Part model, mm, in its own coordinate system. A direction names the side the tool comes from. Round coordinates to 2 decimals unless told otherwise and drop trailing zeros. Order: outer loops, then holes, each group sorted by start corner. A loop starts at its lowest first (then second) coordinate and runs counter-clockwise, first axis right, second up. Notation, with made-up numbers: M 26.5,-4 L 59.5,-4 A36 ccw 59.5,31 Z; hole C -39,20 d7. An arc over 180 degrees is marked long. Write each question's results on one line, items separated by ' | '. Start each with the question number.
1. Band-saw the part on A-A, the plane x = 49. List the corners of the cut face in (y, z).
2. Drop flat-ended pins along their axis: pin 1 Ø8 at (x, z) = (38, 71) entering from +Y; pin 2 Ø1 at (x, y) = (24, -1.5) entering from -Z. Give the stop position or say it passes through.
3. Band-saw the part on D-D, the plane z = 35. List the corners of the cut face in (x, y), then the cut area to 3 significant figures.
4. Band-saw the part on C-C, the plane x = 19. List the corners of the cut face in (y, z), then the cut area to 3 significant figures.
5. Band-saw the part on B-B, the plane z = 19. List the corners of the cut face in (x, y), then the cut area to 3 significant figures.
6. Which spindle directions (+Z, -Z, +X, -X, +Y, -Y) get a long thin tool onto all of the face, cutting with end or side? Do faces 1 (the face through (26.538, 0.371, 111.632)), 2 (the face through (27.28, 0.33, 110.64)). Say none if no direction does.
7. Probe L1, parallel to Z at x = 31.5, y = -1.35; L2, parallel to Y at x = 38, z = 47.5; L3, parallel to Z at x = 14, y = -0.85. List the from-to ranges inside material, lowest first. Write a range as [from, to].
Autodesk Inventor part; units mm, degrees
ref_plane "YZ Plane" through (0, 0, 0) normal (1, 0, 0) x (0, 1, 0)
ref_plane "XZ Plane" through (0, 0, 0) normal (0, 1, 0) x (-1, 0, 0)
ref_plane "XY Plane" through (0, 0, 0) normal (0, 0, 1) x (1, 0, 0)
sketch "Sketch1" plane through (0, 0, 0) normal (0, 0, 1) x (1, 0, 0)
  line L0 (0.222, 0) -> (0.222, -1)
  line L1 (0.222, 0) -> (0.222, -5.0532)
  line L2 (0.222, -1) -> (-0.778, -1)
  line L3 (-0.778, -1) -> (-0.778, -2.2)
  line L4 (53.594, 0) -> (55.372, 0)
  line L5 (53.594, 0) -> (53.594, -1)
  line L6 (53.594, 0) -> (53.594, -17.7031)
  line L7 (53.594, -1) -> (54.594, -1)
  line L8 (54.594, -1) -> (54.594, -2.2)
  line L9 (-1.778, 0) -> (-1.778, -17.5378)
  line L10 (-0.778, -2.2) -> (54.594, -2.2)
  line L11 (0.222, 0) -> (53.372, 0)
  line L12 (0.222, -1) -> (53.594, -1)
  line L13 (-0.778, -2.2) -> (54.594, -2.2)
  line L14 (54.594, -2.2) -> (54.594, -1)
  line L15 (54.594, -1) -> (-0.778, -1)
  line L16 (-0.778, -1) -> (-0.778, -2.2)
  line L17 (-0.278, -2.2) -> (-0.278, -1)
  line L18 (54.094, -2.2) -> (54.094, -1)
  point P0 (0, 0)
  point P1 (26.797, 5.3109)
  dimension "d0" = 1
  dimension "d1" = 1
  dimension "d2" = 1.2
  dimension "d3" = 1
  dimension "d4" = 1
  dimension "d5" = 1.2
extrude "Extrusion1" add sketch "Sketch1" along normal blind 111.76 contours L12 L6 L10 L1 | L1 L10 L17 L2 | L7 L18 L10 L6
sketch "Sketch2" plane through (-0.778, -1, 0) normal (0, 1, 0) x (1, 0, 0)
  line L0 (54.872, 0) -> (0.5, 0)
  line L1 (0, 0) -> (55.372, 0)
  line L2 (27.686, 0) -> (27.686, -25)
  line L3 (27.686, -25) -> (17.686, -25)
  line L4 (17.686, -25) -> (17.686, 0)
  line L5 (27.686, -25) -> (37.686, -25)
  line L6 (37.686, -25) -> (37.686, 0)
  line L7 (17.686, 0) -> (37.686, 0)
  point P0 (0.778, 0)
  dimension "d8" = 25
  dimension "d9" = 10
  dimension "d10" = 10
extrude "Extrusion2" cut sketch "Sketch2" against normal blind 111.76
sketch "Sketch3" plane through (-0.778, -1, 111.76) normal (0, 1, 0) x (1, 0, 0)
  line L0 (0, 111.76) -> (0, 0)
  line L1 (0, 0) -> (1.27, 0)
  line L2 (54.872, 0) -> (0.5, 0)
  line L3 (55.372, 0) -> (54.102, 0)
  line L4 (1.27, 0) -> (54.102, 0)
  line L5 (1.27, 0) -> (1.27, 0.9906)
  line L6 (1.27, 0.9906) -> (54.102, 0.9906)
  line L7 (54.102, 0.9906) -> (54.102, 0)
  point P0 (0.778, 111.76)
  dimension "d13" = 1.27
  dimension "d14" = 1.27
  dimension "d15" = 0.9906
ref_plane "Work Plane3" through (54.594, -1, 111.76) normal (0, -0.9957, 0.0929) x (-1, 0, 0)
ref_plane "Work Plane2" through (-0.778, -2.2, 111.76) normal (0, -0.0929, -0.9957) x (1, 0, 0)
sketch "Sketch5" plane through (54.594, -1, 111.76) normal (0, -0.9957, 0.0929) x (-1, 0, 0)
  line L0 (0, 111.76) -> (0, 0)
  line L1 (0, 0) -> (1.27, 0)
  line L2 (55.372, 0) -> (0, 0)
  line L3 (55.372, 0) -> (54.102, 0)
  line L4 (1.27, 0) -> (54.102, 0)
  line L5 (1.27, 0) -> (1.27, 0.9906)
  line L6 (1.27, 0.9906) -> (54.102, 0.9906)
  line L7 (54.102, 0.9906) -> (54.102, 0)
  point P0 (54.594, 111.1839)
  point P1 (0.778, 111.76)
  dimension "d26" = 1.27
  dimension "d27" = 1.27
  dimension "d28" = 0.9906
extrude "Extrusion5" add sketch "Sketch5" against normal blind 2.794
properties part number "betonbottom"
Solution:
1) outline: M -2.2,0 L -1,0 L -1,110.77 L 1.69,110.51 L 1.78,111.5 L -1,111.76 L -2.2,111.76 Z
2) pin 1: y = -1 | pin 2: z = 25
3) outline: M -0.28,-2.2 L 54.09,-2.2 L 54.09,-1 L -0.28,-1 Z | area: 65.2 mm^2
4) outline: M -2.2,25 L -1,25 L -1,110.77 L 1.69,110.51 L 1.78,111.5 L -1,111.76 L -2.2,111.76 Z | area: 107 mm^2
5) outline: M -0.28,-2.2 L 16.91,-2.2 L 16.91,-1 L -0.28,-1 Z; M 36.91,-2.2 L 54.09,-2.2 L 54.09,-1 L 36.91,-1 Z | area: 41.2 mm^2
6) face 1: +Z, +X, -X, +Y | face 2: -Z, +X, -X
7) L1: [25, 111.76] | L2: [-2.2, -1] | L3: [110.75, 111.75]
